Read the model definition and answer for the solid it produces. Units are mm, in the model's axes. A direction names the side the tool comes from. Coordinates: 2 decimals unless noted, no trailing zeros. Write each loop counter-clockwise with the first axis right and the second up, starting at its lowest first coordinate (ties: lowest second). Pieces come first, ordered by that corner, then holes. Notation, with made-up numbers: (59, 58.5) -> (118, 58.5) arc R21 ccw to (118, 72.5) -> close; hole circle Ø3 at (4, -17.75). An arc over 180 degrees is marked (long way). Use CSV: the item, a comma, the result in double quotes.
Autodesk Inventor part; units mm, degrees
ref_plane "YZ Plane" through (0, 0, 0) normal (1, 0, 0) x (0, 1, 0)
ref_plane "XZ Plane" through (0, 0, 0) normal (0, 1, 0) x (-1, 0, 0)
ref_plane "XY Plane" through (0, 0, 0) normal (0, 0, 1) x (1, 0, 0)
sketch "スケッチ1" plane through (0, 0, 0) normal (0, 0, 1) x (1, 0, 0)
  line L0 (0, 0) -> (10, 0)
  line L1 (10, 0) -> (10, 60)
  line L2 (10, 60) -> (0, 60)
  line L3 (0, 60) -> (0, 0)
  dimension "d0" = 10
  dimension "d1" = 60
extrude "押し出し1" add sketch "スケッチ1" along normal blind 5
sketch "スケッチ3" plane through (0, 0, 5) normal (0, 0, 1) x (1, 0, 0)
  line L0 (10, 0) -> (10, 60)
  line L1 (10, 60) -> (0, 60)
  line L2 (0, 60) -> (0, 0)
  line L3 (0, 0) -> (10, 0)
  line L4 (10, 60) -> (0, 60)
  line L5 (0, 60) -> (0, 0)
  line L6 (0, 0) -> (10, 0)
  line L7 (10, 0) -> (10, 60)
extrude "押し出し2" add sketch "スケッチ3" along normal blind 30
sketch "スケッチ4" plane through (10, 0, 0) normal (1, 0, 0) x (0, 0, -1)
  line L0 (0, 60) -> (-35, 60)
  line L1 (0, 0) -> (0, 60)
  line L2 (0, 0) -> (-35, 0)
  line L3 (-35, 60) -> (-5, 60)
  line L4 (-5, 60) -> (-5, 0)
  line L5 (-5, 0) -> (-35, 0)
  line L6 (-35, 0) -> (-35, 60)
  line L7 (-30, 55) -> (-10, 55)
  line L8 (-10, 55) -> (-10, 5)
  line L9 (-10, 5) -> (-30, 5)
  line L10 (-30, 5) -> (-30, 55)
  dimension "d37" = 5
  dimension "d38" = 5
  dimension "d39" = 20
extrude "押し出し3" cut sketch "スケッチ4" against normal blind 40 contours L7 L8 L9 L10
sketch "スケッチ5" plane through (0, 0, 0) normal (0, 0, -1) x (-1, 0, 0)
  line L0 (0, 60) -> (0, 0)
  line L1 (0, 0) -> (-10, 0)
  point P0 (-5, 50)
  point P1 (-5, 10)
  dimension "d23" = 40
  dimension "d24" = 5
  dimension "d25" = 5
  dimension "d26" = 10
hole "穴2" at (5, 50, 0) at (5, 10, 0) direction (0, 0, 1) diameter 5 depth 8
fillet "フィレット1" radius 2 6 edges at (5, 55, 10) (5, 55, 30) (5, 5, 30) (5, 5, 10) (5, 0, 35) (5, 60, 35)
properties part number "BP_BOX-handle" material "ABS プラスチック"
1. A cutting plane is placed at C-C (x = 6.5). Give the vertices of the cut face in (y, z), and give its area (3 significant figures).
Solutions:
outline,"(0, 0) -> (8, 0) -> (8, 8) -> (12, 8) -> (12, 0) -> (48, 0) -> (48, 8) -> (52, 8) -> (52, 0) -> (60, 0) -> (60, 33) arc R2 ccw to (58, 35) -> (2, 35) arc R2 ccw to (0, 33) -> close; hole (5, 12) arc R2 ccw to (7, 10) -> (53, 10) arc R2 ccw to (55, 12) -> (55, 28) arc R2 ccw to (53, 30) -> (7, 30) arc R2 ccw to (5, 28) -> close"
area,"1,040 mm^2"
2. Find the intervals of material crossed by line 1 along Y through (x, z) = (5, 2.25); line 2 along Z through (x, y) = (5.25, 28); line 3 along Y through (x, z) = (2, 25), in increasing order.
Solutions:
line 1,"y = 0 to 7.5, 12.5 to 47.5, 52.5 to 60"
line 2,"z = 0 to 10, 30 to 35"
line 3,"y = 0 to 5, 55 to 60"
3. A cutting plane is placed at D-D (z = 6.5). Give the vertices of the cut face in (x, y), and give its area (3 significant figures).
Solutions:
outline,"(0, 0) -> (10, 0) -> (10, 60) -> (0, 60) -> close; hole circle Ø5 at (5, 10); hole circle Ø5 at (5, 50)"
area,"561 mm^2"
4. A tool of negligible diameter and unlimited length cuts with its end or side. For faces 1 (the flat face through (5, 30, 10)), 2 (the flat face through (5, 50, 8)), 3 (the cylindrical face through (5.07, 0.6, 34.43)), from which of +Z, -Z, +X, -X, +Y, -Y can it reach the whole face along a straight path? Write none if from no direction.
Solutions:
face 1,"+X, -X"
face 2,"-Z"
face 3,"+Z, +X, -X, -Y"
5. A cutting plane is placed at A-A (z = 26). Give the vertices of the cut face in (x, y).
Solutions:
outline,"(0, 0) -> (10, 0) -> (10, 5) -> (0, 5) -> close; (0, 55) -> (10, 55) -> (10, 60) -> (0, 60) -> close"
6. This flat-tipped pin is pushed along its axis until it touches: pin 1 Ø4 at (x, y) = (4.5, 11) entering from -Z. Where does it stop, or does it pass through?
Solutions:
pin 1,"stops at z = 0"
7. For a pull along Z with two mould halves and no side action, classify faces 4 (the cylindrical face through (4.93, 5.6, 10.57)), 5 (the cylindrical face through (4.93, 59.4, 34.43)), 6 (the cylindrical face through (5.96, 52.31, 4.06)) as pulls with the +Z half, pulls with the -Z half, needs draft (parallel to the pull), parting line crosses it, or undercut.
Solutions:
face 4,"undercut"
face 5,"pulls with the +Z half"
face 6,"needs draft"
8. A cutting plane is placed at B-B (y = 50). Give the vertices of the cut face in (x, z).
Solutions:
outline,"(0, 0) -> (2.5, 0) -> (2.5, 8) -> (7.5, 8) -> (7.5, 0) -> (10, 0) -> (10, 10) -> (0, 10) -> close; (0, 30) -> (10, 30) -> (10, 35) -> (0, 35) -> close"
